Verification items for the finished model (mm, model axes). A direction names the side the tool comes from. Round coordinates to 2 decimals unless told otherwise and drop trailing zeros. Write each loop counter-clockwise with the first axis right and the second up, starting at its lowest first coordinate (ties: lowest second). Pieces come first, ordered by that corner, then holes. Notation, with made-up numbers: M 34,88 L 43,88 A20 cw 43,122 Z; hole C 83,14 d8. An arc over 180 degrees is marked long. One line per item, written item: value. Start each with the question number.
Item 1: Section check A-A, the plane y = 27. Record the cut outline in (x, z).
Item 2: Thickness scan on probe 1 along X at (y, z) = (-18, 3.75); probe 2 along X at (y, z) = (-64, 4.55); probe 3 along Y at (x, z) = (10.5, 4.7). Record the ranges inside material, lowest first. Write a range as from..to.
Item 3: Draft check along Y on faces 6 (the face through (0.11, 50.75, 3.04)), 7 (the face through (-17, 1, 0)), 8 (the face through (35, -80.75, 3)). Enter one of: +Y half, -Y half, draft (parallel to the pull), parting line (faces both ways), or undercut.
Item 4: Section check B-B, the plane x = 0. Record the cut outline in (y, z), then the cut area to 3 significant figures.
Item 5: Tool access check on faces 1 (the face through (-53.5, -71, 3)), 2 (the face through (5, 6, 3)), 3 (the face through (53.5, -71, 3)), 4 (the face through (-15, -70, 3)), 5 (the face through (-1, 80.75, 3)). Record the directions out of +Z, -Z, +X, -X, +Y, -Y that give a thin tool (end or side, any length) a straight path to the whole face; none if there is none.
Item 6: Section check C-C, the plane z = 2.9. Record the cut outline in (x, y).
Item 7: Gauge pin test, flat ends, axial feed: pin 1 (2 mm diameter, centred on x = -1.5, z = 1, fed in from -Y); pin 2 (3 mm diameter, centred on x = -65.5, z = 1.5, fed in from -Y); pin 3 (1.8 mm diameter, centred on y = -68, z = 2.5, fed in from -X); pin 4 (6 mm diameter, centred on x = 21, y = -48, fed in from -Z). Record the tip position at first contact, or that the pin passes through.
Autodesk Inventor part; units mm, degrees
sketch "Sketch1" plane through (0, 0, 0) normal (0, 0, 1) x (1, 0, 0)
  line L0 (-73.5, 80.75) -> (73.5, 80.75)
  line L1 (73.5, 80.75) -> (73.5, -80.75)
  line L2 (73.5, -80.75) -> (-73.5, -80.75)
  line L3 (-73.5, -80.75) -> (-73.5, 80.75)
  point P0 (0, 80.75)
  point P1 (0, 0)
  point P2 (-73.5, 0)
  dimension "d0" = 147
  dimension "d1" = 161.5
extrude "Extrusion1" add sketch "Sketch1" along normal blind 6
sketch "Sketch2" plane through (0, 0, 6) normal (0, 0, 1) x (1, 0, 0)
  line L0 (-73.5, 80.75) -> (-73.5, -80.75)
  line L1 (-73.5, -80.75) -> (-73.5, -60.75)
  line L2 (-53.5, -80.75) -> (-73.5, -80.75)
  line L3 (-73.5, -60.75) -> (-53.5, -60.75)
  line L4 (-53.5, -60.75) -> (-53.5, -80.75)
  line L5 (-73.5, -80.75) -> (73.5, -80.75)
  line L6 (-53.5, -80.75) -> (-73.5, -80.75)
  point P0 (0, 0)
  point P1 (40.5, -62.5)
  dimension "d14" = 20
  dimension "d18" = 20
extrude "Extrusion2" cut sketch "Sketch2" against normal blind 15
mirror "Mirror1" about plane through (0, 0, 0) normal (1, 0, 0) of "Extrusion2"
sketch "Sketch5" plane through (0, 0, 6) normal (0, 0, 1) x (1, 0, 0)
  line L0 (-15, -59.25) -> (15, -59.25)
  line L1 (15, -59.25) -> (15, -80.75)
  line L2 (15, -80.75) -> (-15, -80.75)
  line L3 (-15, -80.75) -> (-15, -59.25)
  line L4 (-53.5, -80.75) -> (53.5, -80.75)
  point P0 (0, 0)
  point P1 (0, -80.75)
  point P2 (0, -80.75)
  point P3 (0, -80.75)
  dimension "d19" = 30
  dimension "d20" = 21.5
extrude "Extrusion4" cut sketch "Sketch5" against normal blind 6
sketch "Sketch3" plane through (0, 0, 6) normal (0, 0, 1) x (1, 0, 0)
  line L0 (-73.5, -80.75) -> (73.5, -80.75)
  line L1 (-15, -59.25) -> (15, -59.25)
  line L2 (0, -80.75) -> (0, -69.25) construction
  line L3 (0, -69.25) -> (0, -44.25) construction
  line L4 (0, -44.25) -> (0, -34.25) construction
  line L5 (-5, 45.75) -> (5, 45.75) construction
  line L6 (5, 45.75) -> (5, -34.25)
  line L7 (5, -34.25) -> (-5, -34.25) construction
  line L8 (-5, -34.25) -> (-5, 45.75)
  arc A0 (-5, -34.25) -> (5, -34.25) centre (0, -34.25) ccw
  arc A1 (5, 45.75) -> (-5, 45.75) centre (0, 45.75) ccw
  line L9 (73.5, 80.75) -> (-73.5, 80.75)
  line L10 (0, 80.75) -> (0, 55.75) construction
  line L11 (0, 55.75) -> (0, 45.75) construction
  point P0 (0, 0)
  point P1 (-40.5, -62.5)
  point P2 (40.5, -62.5)
  point P3 (73.5, -80.75)
  dimension "d23" = 11.5
  dimension "d24" = 25
  dimension "d26" = 10
  dimension "d27" = 10
  dimension "d29" = 25
  dimension "d30" = 10
extrude "Extrusion3" cut sketch "Sketch3" against normal blind 6
fillet "Fillet1" radius 1 12 edges at (-73.5, 80.75, 3) (73.5, 80.75, 3) (73.5, -60.75, 3) (53.5, -60.75, 3) (53.5, -80.75, 3) (15, -80.75, 3) (15, -59.25, 3) (-15, -59.25, 3) (-15, -80.75, 3) (-53.5, -80.75, 3) (-73.5, -60.75, 3) (-53.5, -60.75, 3)
equation "\"d7\" = d5"
properties part number "Hammer_wall" material "MDF Medium Density Fiberboard"
Response values:
1. outline: M -73.5,0 L -5,0 L -5,6 L -73.5,6 Z; M 5,0 L 73.5,0 L 73.5,6 L 5,6 Z
2. probe 1: x = -73.5..-5, 5..73.5
2. probe 2: x = -53.5..-15, 15..53.5
2. probe 3: y = -59.25..80.75
3. face 6: undercut
3. face 7: draft
3. face 8: -Y half
4. outline: M -59.25,0 L -39.25,0 L -39.25,6 L -59.25,6 Z; M 50.75,0 L 80.75,0 L 80.75,6 L 50.75,6 Z
4. area: 300 mm2
5. face 1: +Z, -Z, -X, -Y
5. face 2: +Z, -Z
5. face 3: +Z, -Z, +X, -Y
5. face 4: +Z, -Z, -Y
5. face 5: +Z, -Z, +X, -X, +Y
6. outline: M -73.5,-59.75 A1 ccw -72.5,-60.75 L -54.5,-60.75 A1 cw -53.5,-61.75 L -53.5,-79.75 A1 ccw -52.5,-80.75 L -16,-80.75 A1 ccw -15,-79.75 L -15,-60.25 A1 cw -14,-59.25 L 14,-59.25 A1 cw 15,-60.25 L 15,-79.75 A1 ccw 16,-80.75 L 52.5,-80.75 A1 ccw 53.5,-79.75 L 53.5,-61.75 A1 cw 54.5,-60.75 L 72.5,-60.75 A1 ccw 73.5,-59.75 L 73.5,79.75 A1 ccw 72.5,80.75 L -72.5,80.75 A1 ccw -73.5,79.75 Z; hole M -5,-34.25 A5 ccw 5,-34.25 L 5,45.75 A5 ccw -5,45.75 Z
7. pin 1: stops at y = -59.25
7. pin 2: stops at y = -60.75
7. pin 3: stops at x = -53.5
7. pin 4: stops at z = 0
